Part print with two shaded views. Sizes in mm from the minimum x, y, z corner. Round coordinates to 2 decimals unless told otherwise and drop trailing zeros. Order: outer loops, then holes, each group sorted by start corner. A loop starts at its lowest first (then second) coordinate and runs counter-clockwise, first axis right, second up. Notation, with made-up numbers: M -8.75,64 L 5.25,64 A11 cw 5.25,77 Z; hole C -21.75,16 d6. An arc over 180 degrees is marked long. Return JSON: item names as keys, results as strings. Group by question number.
Item 1: Slice it at A-A on y = 2.65. Write the cut outline in (x, z).
Item 2: Slice it at D-D on x = 33. Write the cut outline in (y, z), then the cut area to 3 significant figures.
Item 3: Slice it at B-B on x = 6.5. Write the cut outline in (y, z) (1 decimal).
Item 4: Pin check, flat tip, straight feed: pin 1 Ø6 at (x, z) = (39.5, 69.5) entering from +Y. Stop position of the tip, or through.
Item 5: Probe line 1 along X through (y, z) = (3.35, 20); line 2 along Z through (x, y) = (34, 2.15); line 3 along X through (y, z) = (2.05, 30.5). List the from-to ranges inside material, lowest first.
Item 6: Pull direction Z, two halves, no side cores. Call the marked faces 1 and 2: pulls with the +Z half, pulls with the -Z half, needs draft (parallel to the pull), parting line crosses it, or undercut.
Item 7: Slice it at C-C on z = 38.5. Write the cut outline in (x, y).
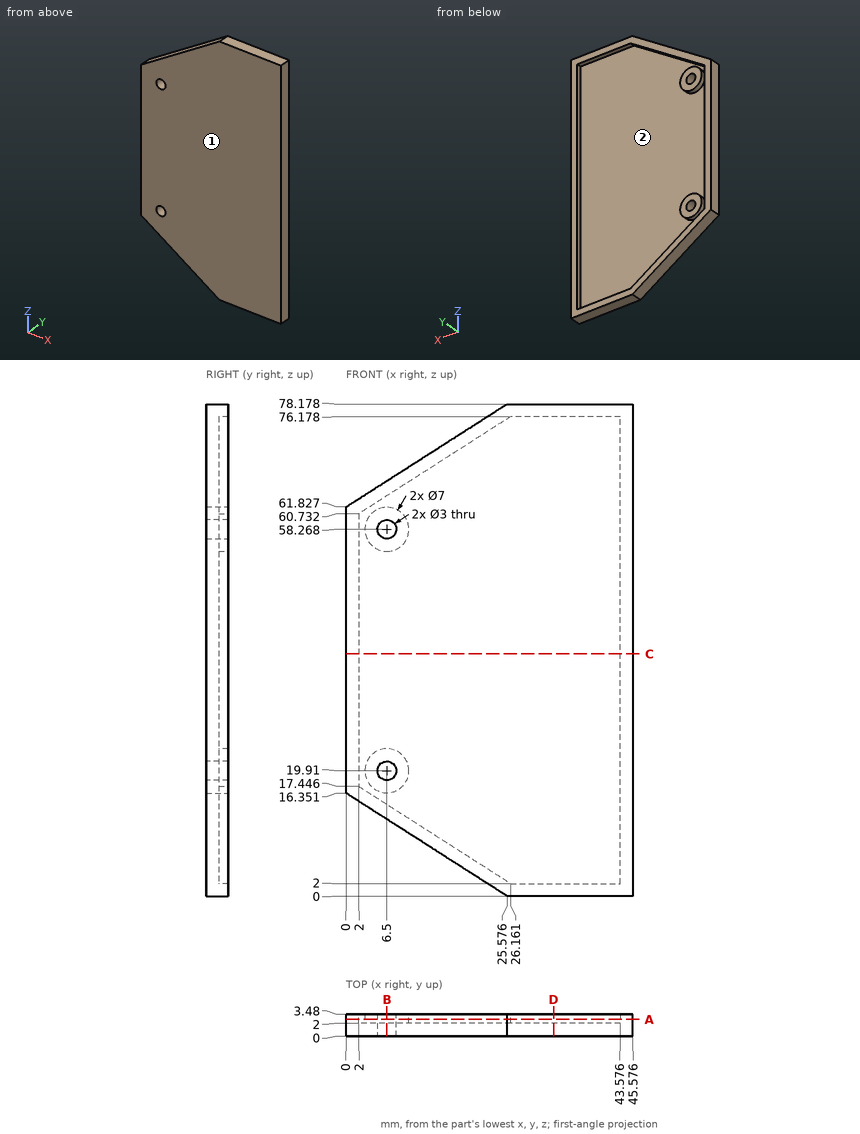
Output values:
{
 "1": {"outline": "M 0,16.35 L 25.58,0 L 45.58,0 L 45.58,78.18 L 25.58,78.18 L 0,61.83 Z; C 6.5,19.91 d7; C 6.5,58.27 d7; hole M 2,17.45 L 26.16,2 L 43.58,2 L 43.58,76.18 L 26.16,76.18 L 2,60.73 Z; hole C 6.5,19.91 d3; hole C 6.5,58.27 d3"},
 "2": {"outline": "M 0,0 L 3.48,0 L 3.48,2 L 2,2 L 2,76.18 L 3.48,76.18 L 3.48,78.18 L 0,78.18 Z", "area": "162 mm²"},
 "3": {"outline": "M 0,12.2 L 3.5,12.2 L 3.5,14.6 L 2,14.6 L 2,16.4 L 3.5,16.4 L 3.5,18.4 L 0,18.4 Z; M 0,21.4 L 3.5,21.4 L 3.5,23.4 L 2,23.4 L 2,54.8 L 3.5,54.8 L 3.5,56.8 L 0,56.8 Z; M 0,59.8 L 3.5,59.8 L 3.5,61.8 L 2,61.8 L 2,63.6 L 3.5,63.6 L 3.5,66 L 0,66 Z"},
 "4": {"pin 1": "y = 2"},
 "5": {"line 1": "0 to 2, 3 to 5, 8 to 10, 43.58 to 45.58", "line 2": "0 to 2, 76.18 to 78.18", "line 3": "0 to 2, 43.58 to 45.58"},
 "6": {"face 1": "needs draft", "face 2": "undercut"},
 "7": {"outline": "M 0,0 L 45.58,0 L 45.58,3.48 L 43.58,3.48 L 43.58,2 L 2,2 L 2,3.48 L 0,3.48 Z"}
}
